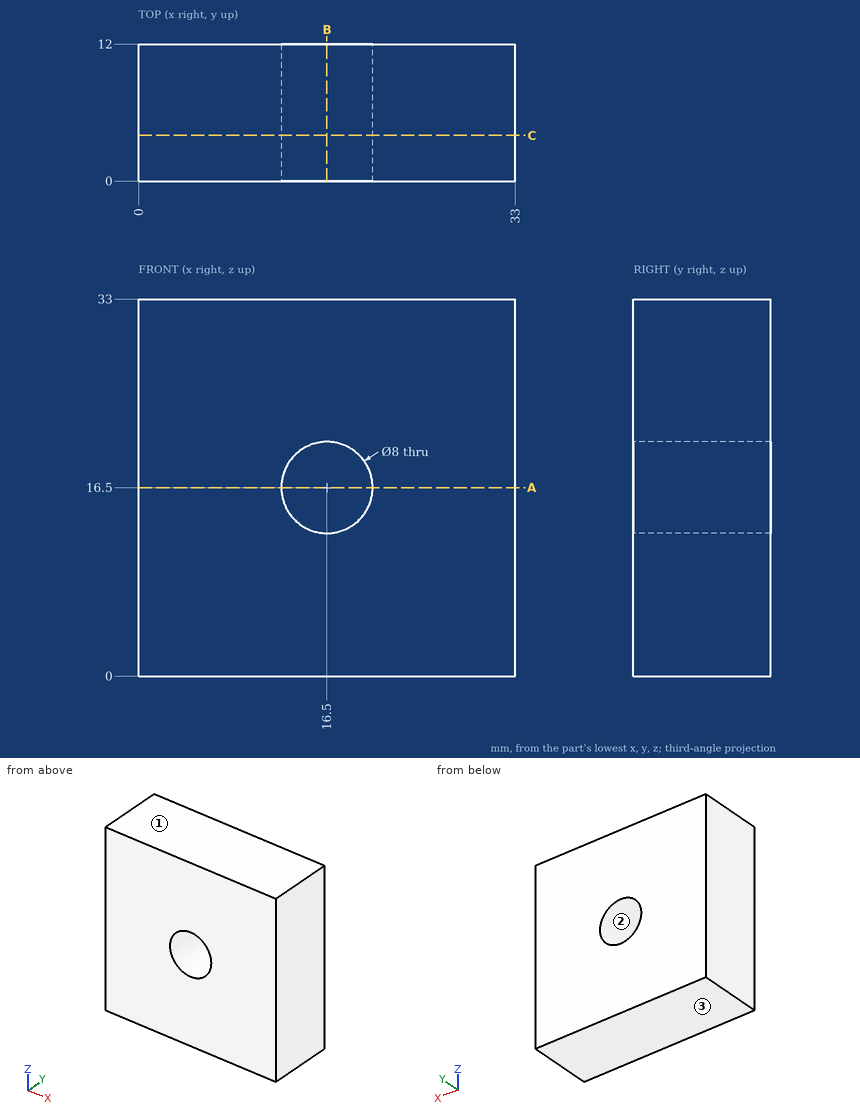
Could you check a few things on this drawing? It's one solid part, dimensions in mm from its lowest x, y, z. Give positions to 0.01 mm unless a question says otherwise; leave off trailing zeros. Order: outer loops, then holes, each group sorted by start corner. A loop starts at its lowest first (then second) coordinate and runs counter-clockwise, first axis right, second up. Notation, with made-up numbers: (34, -5) - (87, -5) arc R30 cw to (87, 19) - close; hole circle Ø3 at (6.25, -15.75). An arc over 180 degrees is marked (long way). Return JSON: item names as keys, results as strings. Group by question number.
Q1. Please list where these lines run through material, in increasing order: line 1 along Z through (x, y) = (16.5, 5); line 2 along Z through (x, y) = (20, 11.5); line 3 along X through (y, z) = (11.25, 15). Write a range as [from, to].
Q2. Suppose I cut it at C-C, the plane y = 4. Please give me the cut outline in (x, z).
Q3. Suppose I cut it at A-A, the plane z = 16.5. Please give me the cut outline in (x, y), and give its area (3 significant figures).
Q4. Suppose I cut it at B-B, the plane x = 16.5. Please give me the cut outline in (y, z).
Q5. Will this pin go through, and if not, where does the flat tip stop? pin 1 Ø8 at (x, z) = (23.5, 27.5) entering from -Y.
Q6. Thinking about a two-plate mould opening in Z: for the marked faces 1, 2 and 3, which applies, pulls with the +Z half, pulls with the -Z half, needs draft (parallel to the pull), parting line crosses it, or undercut?
Resolved:
{
 "1": {"line 1": "z = [0, 12.5], [20.5, 33]", "line 2": "z = [0, 14.56], [18.44, 33]", "line 3": "x = [0, 12.79], [20.21, 33]"},
 "2": {"outline": "(0, 0) - (33, 0) - (33, 33) - (0, 33) - close; hole circle Ø8 at (16.5, 16.5)"},
 "3": {"outline": "(0, 0) - (12.5, 0) - (12.5, 12) - (0, 12) - close; (20.5, 0) - (33, 0) - (33, 12) - (20.5, 12) - close", "area": "300 mm2"},
 "4": {"outline": "(0, 0) - (12, 0) - (12, 12.5) - (0, 12.5) - close; (0, 20.5) - (12, 20.5) - (12, 33) - (0, 33) - close"},
 "5": {"pin 1": "stops at y = 0"},
 "6": {"face 1": "pulls with the +Z half", "face 2": "undercut", "face 3": "pulls with the -Z half"}
}
